Here's how the part is built. I have some questions about the finished solid (model axes, mm). A direction names the side the tool comes from. Give positions to 0.01 mm unless a question says otherwise; leave off trailing zeros. Write each loop counter-clockwise with the first axis right and the second up, starting at its lowest first coordinate (ties: lowest second). Pieces come first, ordered by that corner, then holes. Notation, with made-up numbers: (78, 6) -> (134, 6) arc R17 ccw to (134, 20) -> close; hole circle Ø8 at (28, 9.25). An arc over 180 degrees is marked (long way). Answer as CSV lines item,"result". Start each with the question number.
from build123d import *

# Parameters (mm, degrees)
F0_R             = 6
F0_R_2           = 3.975
F1_DEPTH         = 15.25
F2_R             = 6
F2_R_2           = 3.975
F3_DEPTH         = 6.25
F4_R             = 3.975
F5_DEPTH         = 4
F6_R             = 1.5
F7_DEPTH         = 4.5
F8_R             = 1.75
F9_DEPTH         = 15.251
F10_R            = 1
F11_DEPTH        = 15.251
F11_COPIES_COUNT = 2
F11_COPIES_PITCH = 22.388613
F12_R            = 1.7592557298
F12_R_2          = 1
F12_R_3          = 1.75
F13_DEPTH        = 8
F14_R            = 2.1
F15_DEPTH        = 8
F17_DEPTH        = 2
F18_R            = 1.6
F19_DEPTH        = 12
F20_R            = 0.9
F21_DEPTH        = 20
F23_DEPTH        = 15.25
F24_R            = 1.5
F25_DEPTH        = 11


# Not quite as in the source:
# - a pattern or mirror of a feature is missing from the dataset's text; its kind, count and spacing are read off the source's solid
# - a feature names something its author has since deleted; it is built from what else it names


with BuildPart() as f1:
    # F0 (on Front) → F1 (new body)
    with BuildSketch(Plane.XZ):
        with BuildLine():
            Line((-14.75, -13.5), (14.75, -13.5))
            ThreePointArc((14.75, -13.5), (15.4571067812, -13.2071067812), (15.75, -12.5))
            Line((15.75, -12.5), (15.75, 12.5))
            ThreePointArc((15.75, 12.5), (15.4571067812, 13.2071067812), (14.75, 13.5))
            Line((14.75, 13.5), (-14.75, 13.5))
            ThreePointArc((-14.75, 13.5), (-15.4571067812, 13.2071067812), (-15.75, 12.5))
            Line((-15.75, 12.5), (-15.75, -12.5))
            ThreePointArc((-15.75, -12.5), (-15.4571067812, -13.2071067812), (-14.75, -13.5))
        make_face()
        Circle(F0_R, mode=Mode.SUBTRACT)
        Circle(F0_R)
        Circle(F0_R_2, mode=Mode.SUBTRACT)
    extrude(amount=F1_DEPTH)

    # F2 (on face) → F3 (cut)
    with BuildSketch(Plane(origin=(0, 0, 0), x_dir=(-1, 0, 0), z_dir=(0, 1, 0))):
        Circle(F2_R)
        Circle(F2_R_2, mode=Mode.SUBTRACT)
    extrude(amount=-F3_DEPTH, mode=Mode.SUBTRACT)

    # F4 (on face) → F5 (cut)
    with BuildSketch(Plane.XZ.offset(15.25)):
        with BuildLine():
            Line((-2.2497879514, -4.6444608866), (-2.2497871292, -3.8972372103))
            ThreePointArc((-2.2497871292, -3.8972372103), (4.5, -4.9516e-06), (-2.2497785524, 3.8972421615))
            Line((-2.2497785524, 3.8972421615), (-2.2497777241, 4.6499983495))
            ThreePointArc((-2.2497777241, 4.6499983495), (-3.7497777241, 6.15), (-5.2497777241, 4.6499983495))
            Line((-5.2497777241, 4.6499983495), (-5.2497768955, 3.8969854991))
            ThreePointArc((-5.2497768955, 3.8969854991), (-12, -4.9516e-06), (-5.2497683193, -3.8969805469))
            Line((-5.2497683193, -3.8969805469), (-5.2497674968, -4.6444608866))
            ThreePointArc((-5.2497674968, -4.6444608866), (-5.2497777241, -4.6500016505), (-5.2497674846, -4.6555424145))
            ThreePointArc((-5.2497674846, -4.6555424145), (-3.7497777241, -6.15), (-2.2497879636, -4.6555424145))
            ThreePointArc((-2.2497879636, -4.6555424145), (-2.2497777241, -4.6500016505), (-2.2497879514, -4.6444608866))
        make_face()
        Circle(F4_R, mode=Mode.SUBTRACT)
    extrude(amount=-F5_DEPTH, mode=Mode.SUBTRACT)

    # F6 (on face) → F7 (cut)
    with BuildSketch(Plane.XZ.offset(11.25)):
        with Locations((-7.5, 0)):
            Circle(F6_R)
    extrude(amount=-F7_DEPTH, mode=Mode.SUBTRACT)

    # F8 (on face) → F9 (cut, through all)
    with BuildSketch(Plane(origin=(0, 0, 0), x_dir=(-1, 0, 0), z_dir=(0, 1, 0))):
        with Locations((0, -11)):
            Circle(F8_R)
    f9 = extrude(amount=-F9_DEPTH, mode=Mode.SUBTRACT)

    # F9_copies: F9 across plane
    add(f9.mirror(Plane.XY), mode=Mode.SUBTRACT)

    # F10 (on face) → F11 (cut, through all)
    with BuildSketch(Plane(origin=(0, 0, 0), x_dir=(-1, 0, 0), z_dir=(0, 1, 0))):
        with Locations((-10.5, 0)):
            Circle(F10_R)
        with Locations((10, -9)):
            Circle(F10_R)
    f11 = extrude(amount=-F11_DEPTH, mode=Mode.SUBTRACT)

    # F11_copies: F11 ×2
    with Locations(*[Vector(-0.9156440302, 0, 0.401990062) * (i * F11_COPIES_PITCH) for i in range(1, F11_COPIES_COUNT)]):
        add(f11, mode=Mode.SUBTRACT)

    # F12 (on face) → F13 (cut)
    with BuildSketch(Plane(origin=(0, 0, 0), x_dir=(-1, 0, 0), z_dir=(0, 1, 0))):
        with Locations((10, -9)):
            Circle(F12_R)
        with Locations((10, -9)):
            Circle(F12_R_2, mode=Mode.SUBTRACT)
        with Locations((-10.5, 0)):
            Circle(F12_R_3)
        with Locations((-10.5, 0)):
            Circle(F12_R_2, mode=Mode.SUBTRACT)
        with Locations((10, 9)):
            Circle(F12_R_3)
        with Locations((9.9999998377, 8.9999999288)):
            Circle(F12_R_2, mode=Mode.SUBTRACT)
    extrude(amount=-F13_DEPTH, mode=Mode.SUBTRACT)

    # F14 (on face) → F15 (cut)
    with BuildSketch(Plane.XY.offset(13.5)):
        with Locations((5, -9.75)):
            Circle(F14_R)
    extrude(amount=-F15_DEPTH, mode=Mode.SUBTRACT)

    # F16 (on face) → F17 (cut)
    with BuildSketch(Plane.XZ.offset(11.25)):
        with BuildLine():
            ThreePointArc((-5.2497777241, 4.6499983495), (-3.7497768988, 3.15), (-2.2497777241, 4.65))
            ThreePointArc((-2.2497777241, 4.65), (-3.7497785494, 6.15), (-5.2497777241, 4.6499983495))
        make_face()
    extrude(amount=-F17_DEPTH, mode=Mode.SUBTRACT)

    # F18 (on face) → F19 (cut)
    with BuildSketch(Plane.YZ.offset(15.75)):
        with Locations((-9.75, 7.5)):
            Circle(F18_R)
    extrude(amount=-F19_DEPTH, mode=Mode.SUBTRACT)

    # F20 (on face) → F21 (cut)
    with BuildSketch(Plane.YZ.offset(15.75)):
        with Locations((-9.75, 7.5)):
            Circle(F20_R)
    extrude(amount=-F21_DEPTH, mode=Mode.SUBTRACT)

    # F22 (on face) → F23 (join, through all)
    with BuildSketch(Plane.XZ.offset(15.25)):
        with BuildLine():
            Line((-0.6199523885, 17.1813922581), (-14.75, 13.5))
            Line((-14.75, 13.5), (14.75, 13.5))
            ThreePointArc((14.75, 13.5), (15.4571067812, 13.2071067812), (15.75, 12.5))
            Line((15.75, 12.5), (15.75, 17.3429124444))
            Line((15.75, 17.3429124444), (0.6406479022, 17.3429124444))
            ThreePointArc((0.6406479022, 17.3429124444), (0.005194941, 17.3023680128), (-0.6199523885, 17.1813922581))
        make_face()
    extrude(amount=-F23_DEPTH)

    # F24 (on face) → F25 (cut)
    with BuildSketch(Plane(origin=(-4.2312468171, 0, 16.240518475), x_dir=(0.9676959627, 0, 0.2521200581), z_dir=(-0.2521200581, 0, 0.9676959627))):
        with Locations((-2.4117373396, -9.9919419736)):
            Circle(F24_R)
    extrude(amount=-F25_DEPTH, mode=Mode.SUBTRACT)


solid = f1.part
Item 1: If I drill on line 1 (Z direction, x = 10.5, y = -0.5); line 2 (Z direction, x = -10, y = -12.25); line 3 (Z direction, x = 0.5, y = -9.75), over which ranges is the centre line in solid material (lowest first)? Write a range as [from, to].
Item 2: If we section it at B-B (y = -2.25): Please give me the cut outline in (x, z).
Item 3: If we section it at D-D (z = -12): Please give me the cut outline in (x, y), and give its area (3 significant figures).
Item 4: We'd pull the mould along X, two halves only. Please class faces 1 (the face through (15.75, -8, 2)), 2 (the face through (-4, -9.25, 4)), 3 (the face through (-15.465, -7.518, -13.199)): released by +X, released by -X, zero draft, split by the parting line, or undercut.
Item 5: If we section it at C-C (x = 0): Please give me the cut outline in (y, z) (3 decimals).
Item 6: For faces 4 (the face through (-11, -8, 8)), 5 (the face through (-0.14, -9.87, 8.39)), 6 (the face through (5, -10, 5.5)), which set-ups out of +Z, -Z, +X, -X, +Y, -Y let a thin tool reach every point of the face, with its end or its side?
Item 7: If we section it at A-A (z = 0): Please give me the cut outline in (x, y) (3 decimals).
Item 8: I'm going to push flat-ended pins straight in: pin 1 (1.2 mm diameter, centred on x = -10, z = -9, fed in from +Y); pin 2 (2.5 mm diameter, centred on x = 10.5, z = 0, fed in from +Y); pin 3 (0.9 mm diameter, centred on x = -7, z = 0, fed in from -Y); pin 4 (2.5 mm diameter, centred on x = -3.75, z = 4.65, fed in from -Y). Where does each tip first touch, or does it pass through?
Final values:
1,line 1,"[-13.5, -1.75], [1.75, 17.34]"
1,line 2,"[-13.5, -10], [-8, -3.74], [3.74, 8], [10, 14.74]"
1,line 3,"[-13.5, -12.68], [-9.32, -3.94], [3.94, 6.6], [8.4, 9.32], [12.68, 17.34]"
2,outline,"(-15.75, -12.5) arc R1 ccw to (-14.75, -13.5) -> (14.75, -13.5) arc R1 ccw to (15.75, -12.5) -> (15.75, 17.34) -> (0.64, 17.34) arc R5 ccw to (-0.62, 17.18) -> (-14.75, 13.5) arc R1 ccw to (-15.75, 12.5) -> close; hole circle Ø3.52 at (-10, -9); hole circle Ø3.5 at (-10, 9); hole circle Ø12 at (0, 0); hole circle Ø3.5 at (0, -11); hole circle Ø3.5 at (0, 11); hole circle Ø3.5 at (10.5, 0)"
3,outline,"(-15.75, -15.25) -> (-1.44, -15.25) -> (-1.44, 0) -> (-15.75, 0) -> close; (1.44, -15.25) -> (15.75, -15.25) -> (15.75, 0) -> (1.44, 0) -> close"
3,area,"437 mm2"
4,face 1,"released by +X"
4,face 2,"undercut"
4,face 3,"released by -X"
5,outline,"(-15.25, -13.5) -> (0, -13.5) -> (0, -12.75) -> (-15.25, -12.75) -> close; (-15.25, -9.25) -> (0, -9.25) -> (0, -6) -> (-6.25, -6) -> (-6.25, -3.975) -> (-11.25, -3.975) -> (-11.25, -4.5) -> (-15.25, -4.5) -> close; (-15.25, 4.5) -> (-11.25, 4.5) -> (-11.25, 3.975) -> (-6.25, 3.975) -> (-6.25, 6) -> (0, 6) -> (0, 9.25) -> (-15.25, 9.25) -> close; (-15.25, 12.75) -> (0, 12.75) -> (0, 17.302) -> (-15.25, 17.302) -> close; hole circle Ø1.8 at (-9.75, 7.5)"
6,face 4,"+Y"
6,face 5,"+X"
6,face 6,"none"
7,outline,"(-15.75, -15.25) -> (-12, -15.25) -> (-12, -11.25) -> (-9, -11.25) -> (-9, -6.75) -> (-6, -6.75) -> (-6, -11.25) -> (-3.975, -11.25) -> (-3.975, -6.25) -> (-6, -6.25) -> (-6, 0) -> (-15.75, 0) -> close; (3.975, -11.25) -> (4.5, -11.25) -> (4.5, -15.25) -> (9.5, -15.25) -> (9.5, -8) -> (8.75, -8) -> (8.75, 0) -> (6, 0) -> (6, -6.25) -> (3.975, -6.25) -> close; (11.5, -15.25) -> (15.75, -15.25) -> (15.75, 0) -> (12.25, 0) -> (12.25, -8) -> (11.5, -8) -> close"
8,pin 1,"through"
8,pin 2,"y = -8"
8,pin 3,"y = -6.75"
8,pin 4,"y = -9.25"
